Job drawing, mm, ordinate dimensions from the low corner. One solid piece. A direction names the side the tool comes from. Give positions to 0.01 mm unless a question says otherwise; leave off trailing zeros. Order: outer loops, then holes, each group sorted by start corner. A loop starts at its lowest first (then second) coordinate and runs counter-clockwise, first axis right, second up. Notation, with made-up numbers: (42, 77.25) -> (68, 77.25) arc R16 cw to (68, 96.25) -> close; hole circle Ø7 at (-9, -13). An arc over 180 degrees is marked (long way). Use CSV: the item, a comma, the result in double quotes. Start each with the question number.
1. 3-axis set-ups, long thin cutter, end or side, ignore diameter. For the marked faces 1 and 2: which of +Z, -Z, +X, -X, +Y, -Y reach the whole face in a straight line?
2. Cut at A-A on x = 80. List the corners of the cut face in (y, z), then the cut area to 3 significant figures.
3. Drop flat-ended pins along their axis: pin 1 (1.8 mm diameter, centred on x = 15, y = 80, fed in from -Z); pin 2 (1 mm diameter, centred on x = 89.5, z = 64.5, fed in from -Y); pin 3 (12 mm diameter, centred on x = 88.5, y = 78.5, fed in from -Z). Give the stop position or say it passes through.
4. Cut at D-D on z = 72. List the corners of the cut face in (x, y).
5. Wall check: line 1 (Z direction, x = 80, y = 108); line 2 (Y direction, x = 15, z = 90.8); line 3 (X direction, y = 80, z = 92.15). Give the ranges that are in metal, low to high. Write a range as from..to.
6. Cut at B-B on x = 109.5. List the corners of the cut face in (y, z), then the cut area to 3 significant figures.
7. Cut at C-C on y = 35. List the corners of the cut face in (x, z), then the cut area to 3 significant figures.
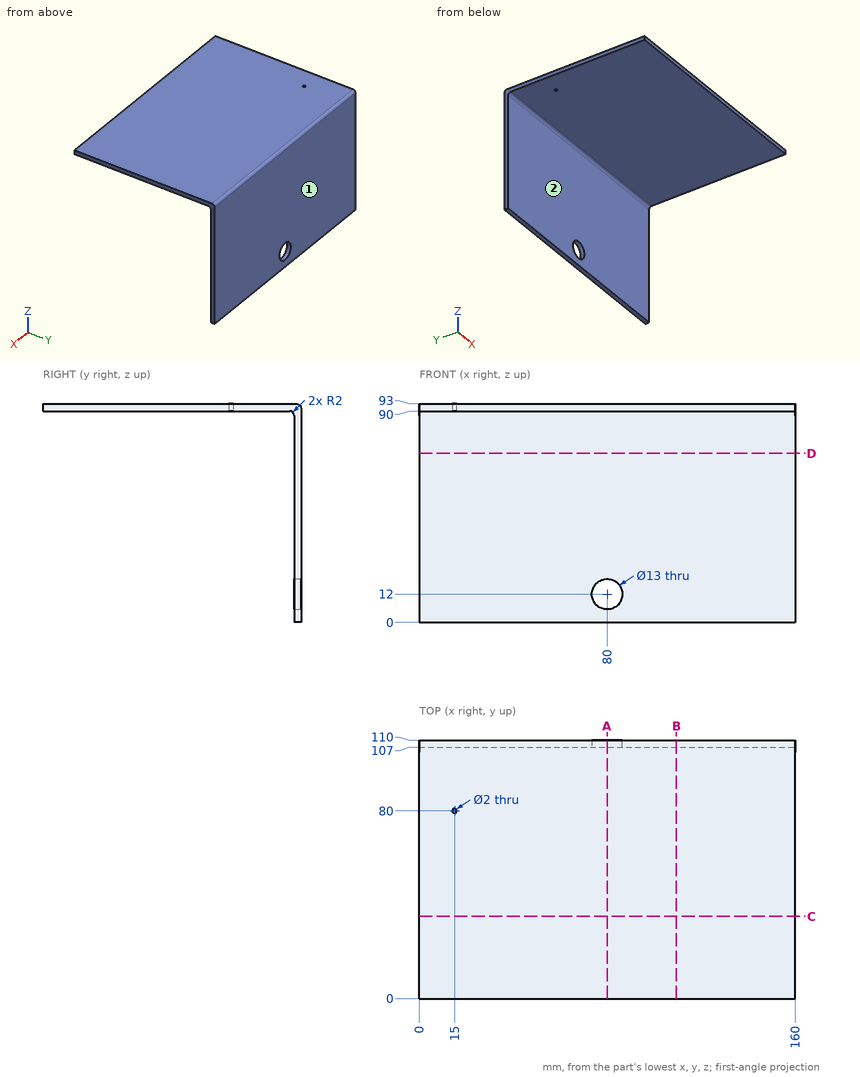
Verdict:
1,face 1,"+Z, -Z, +X, -X, +Y"
1,face 2,"-Z, +X, -X, -Y"
2,outline,"(0, 90) -> (105, 90) arc R2 cw to (107, 88) -> (107, 18.5) -> (110, 18.5) -> (110, 91) arc R2 ccw to (108, 93) -> (0, 93) -> close; (107, 0) -> (110, 0) -> (110, 5.5) -> (107, 5.5) -> close"
2,area,"561 mm^2"
3,pin 1,"through"
3,pin 2,"y = 107"
3,pin 3,"z = 90"
4,outline,"(0, 107) -> (160, 107) -> (160, 110) -> (0, 110) -> close"
5,line 1,"0..5.5, 18.5..93"
5,line 2,"0..79, 81..110"
5,line 3,"0..14, 16..160"
6,outline,"(0, 90) -> (105, 90) arc R2 cw to (107, 88) -> (107, 0) -> (110, 0) -> (110, 91) arc R2 ccw to (108, 93) -> (0, 93) -> close"
6,area,"600 mm^2"
7,outline,"(0, 90) -> (160, 90) -> (160, 93) -> (0, 93) -> close"
7,area,"480 mm^2"
